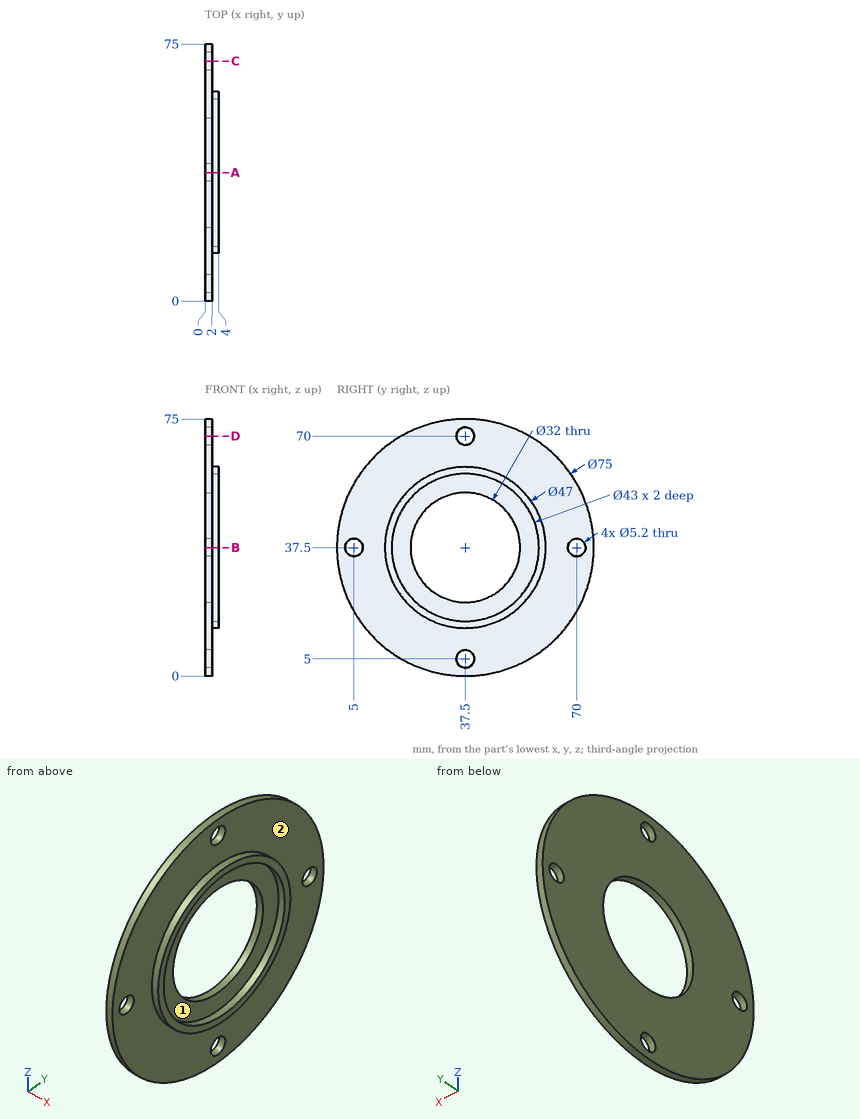
Source: three-view drawing plus pictorial views. Frame: mm from the lowest corner of the part. Give positions to 0.01 mm unless a question says otherwise; leave off trailing zeros. Order: outer loops, then holes, each group sorted by start corner. A loop starts at its lowest first (then second) coordinate and runs counter-clockwise, first axis right, second up. Notation, with made-up numbers: M -9.5,88.25 L 35.5,88.25 A29 cw 35.5,119.25 Z; hole C -39,7.25 d9. An arc over 180 degrees is marked long. One line per question, with ' | ' between items.
1) Section C-C on y = 70. Output: boundary loops of the cut face in (x, z), and give its area (3 significant figures).
Filled in:
outline: M 0,18.79 L 2,18.79 L 2,34.9 L 0,34.9 Z; M 0,40.1 L 2,40.1 L 2,56.21 L 0,56.21 Z | area: 64.4 mm2
2) Draft query along Z for the marked faces 1 and 2. Return one class per face: pulls with the +Z half, pulls with the -Z half, needs draft (parallel to the pull), parting line crosses it, or undercut.
Filled in:
face 1: undercut | face 2: needs draft
3) Contact query for flat-ended pins moving along their axis: P1, Ø8, axis at y = 50.5, z = 9, coming from the +X side; P2, Ø2, axis at x = 1.5, z = 58.5, coming from the +Y side. Output: stop coordinate, or through.
Filled in:
P1: stops at x = 2 | P2: stops at y = 69.22
4) Ray query, L1, parallel to X at y = 52, z = 57.5; L2, parallel to Z at x = 0.25, y = 38; L3, parallel to Z at x = 1.95, y = 47.5. Return the intervals inside material, ascending.
Filled in:
L1: x = 0 to 2 | L2: z = 0 to 2.45, 7.55 to 21.51, 53.49 to 67.45, 72.55 to 75 | L3: z = 1.36 to 25.01, 49.99 to 73.64
5) Section A-A on y = 37.5. Output: boundary loops of the cut face in (x, z), and give its area (3 significant figures).
Filled in:
outline: M 0,0 L 2,0 L 2,2.4 L 0,2.4 Z; M 0,7.6 L 2,7.6 L 2,14 L 4,14 L 4,16 L 2,16 L 2,21.5 L 0,21.5 Z; M 0,53.5 L 2,53.5 L 2,59 L 4,59 L 4,61 L 2,61 L 2,67.4 L 0,67.4 Z; M 0,72.6 L 2,72.6 L 2,75 L 0,75 Z | area: 73.2 mm2
